CAD build for the part. Positions are in the model's coordinates, mm. A direction names the side the tool comes from. Round coordinates to 2 decimals unless told otherwise and drop trailing zeros. Write each loop counter-clockwise with the first axis right and the second up, starting at its lowest first coordinate (ties: lowest second). Pieces come first, ordered by that corner, then holes. Notation, with made-up numbers: (15.25, 8.5) - (31.25, 8.5) arc R19 cw to (31.25, 34.5) - close; hole circle Ø5 at (82, 49). An arc over 180 degrees is marked (long way). Answer in a Markdown table with one row per item.
```python
from build123d import *

# Parameters (mm, degrees)
SKETCH_1_R      = 1.4
EXTRUDE_1_DEPTH = 25
SKETCH_2_W      = 0.5
SKETCH_2_H      = 16
FILLET_1_R      = 0.5


with BuildPart() as part:
    # 草图1 → 凸台-拉伸1 (new body)
    with BuildSketch(Plane(origin=(0, 0, 0), x_dir=(1, 0, 0), z_dir=(0, 1, 0))):
        Circle(SKETCH_1_R)
    extrude(amount=EXTRUDE_1_DEPTH)

    # 草图2 → 切除-旋转1 (revolve, cut)
    with BuildSketch(Plane(origin=(0, 0, 0), x_dir=(0, 0, -1), z_dir=(1, 0, 0))):
        with Locations((1.15, 8)):
            Rectangle(SKETCH_2_W, SKETCH_2_H)
    revolve(axis=Axis((0, 0, 0), (0, -1, 0)), mode=Mode.SUBTRACT)

    # 圆角1
    fillet_1_edges = [part.edges().sort_by_distance(p)[0] for p in [
        (-1.4, 25, 0),
        (0, 0, 0.9),
    ]]
    fillet(fillet_1_edges, radius=FILLET_1_R)


solid = part.part
```
Q1. 3-axis set-ups, long thin cutter, end or side, ignore diameter. For faces 1 (the cylindrical face through (1.335, 20.19, -0.421)), 2 (the cylindrical face through (0.27, 8.36, -0.86)): which of +Z, -Z, +X, -X, +Y, -Y reach the whole face in a straight line?
Computed:
| item | result |
|---|---|
| face 1 | +Y, -Y |
| face 2 | -Y |
Q2. Drill centre lines: line 1 (X direction, y = 8.5, z = 0.1); line 2 (Y direction, x = 0.65, z = 0.7). Where is each one in solid material? Low to high.
Computed:
| item | result |
|---|---|
| line 1 | x = -0.89 to 0.89 |
| line 2 | y = 16 to 25 |
Q3. Flat gauge pin, fed straight in: pin 1 (1.5 mm diameter, centred on x = -1, y = 13.5, fed in from +Z). Where does the tip first touch, or does it go through?
Computed:
| item | result |
|---|---|
| pin 1 | stops at z = 0.86 |
Q4. Saw through at A-A on y = 22.25. List the corners of the cut face in (x, z), then the cut area to 3 significant figures.
Computed:
| item | result |
|---|---|
| outline | circle Ø2.8 at (0, 0) |
| area | 6.16 mm2 |
Q5. Saw through at B-B on y = 2. List the corners of the cut face in (x, z), then the cut area to 3 significant figures.
Computed:
| item | result |
|---|---|
| outline | circle Ø1.8 at (0, 0) |
| area | 2.54 mm2 |
